Job drawing, mm, ordinate dimensions from the low corner. One solid piece. Give positions to 0.01 mm unless a question says otherwise; leave off trailing zeros. Order: outer loops, then holes, each group sorted by start corner. A loop starts at its lowest first (then second) coordinate and runs counter-clockwise, first axis right, second up. Notation, with made-up numbers: M -32,-3.75 L 18,-3.75 A30 cw 18,25.25 Z; hole C 56.25,56.25 d4. An arc over 180 degrees is marked long. Use CSV: the item, a comma, the result in double quotes. Start each with the question number.
Item 1: Two-plate mould, pull along X, no slides. Class the marked faces 1, 2 and 3: pulls with the +X half, pulls with the -X half, needs draft (parallel to the pull), parting line crosses it, or undercut.
Item 2: Band-saw the part on B-B on y = 30. Write the cut outline in (x, z).
Item 3: Wall check: line 1 along Y through (x, z) = (30, 22); line 2 along X through (y, z) = (30.5, 27); line 3 along X through (y, z) = (39, 14). Give the ranges that are in metal, low to high.
Item 4: Pin check, flat tips, straight feed: P1, Ø10, axis at y = 49, z = 7.5, coming from the +X side; P2, Ø6, axis at x = 29.5, z = 23.5, coming from the +Y side; P3, Ø6, axis at x = 52, z = 5, coming from the +Y side; P4, Ø1.5, axis at x = 50.5, y = 53.5, coming from the -Z side. Stop position of each tip, or through.
Item 5: Band-saw the part on A-A on x = 30. Write the cut outline in (y, z), plus the area to 3 significant figures.
Item 6: Band-saw the part on C-C on z = 38.5. Write the cut outline in (x, y).
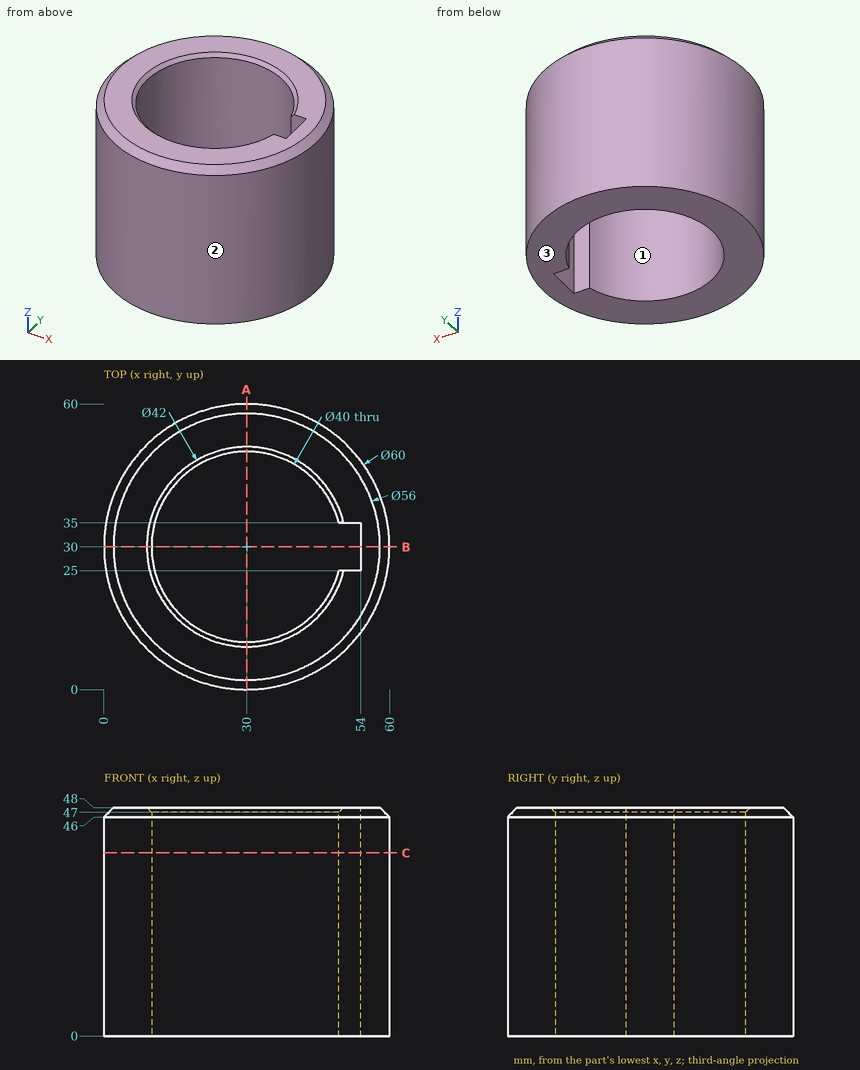
Model answer:
1,face 1,"undercut"
1,face 2,"parting line crosses it"
1,face 3,"needs draft"
2,outline,"M 0,0 L 10,0 L 10,47 L 9,48 L 2,48 L 0,46 Z; M 54,0 L 60,0 L 60,46 L 58,48 L 54,48 Z"
3,line 1,"y = 0 to 10, 50 to 60"
3,line 2,"x = 0 to 10.01, 54 to 60"
3,line 3,"x = 1.38 to 12.14, 47.86 to 58.62"
4,P1,"stops at x = 56.53"
4,P2,"stops at y = 60"
4,P3,"stops at y = 53.22"
4,P4,"passes through"
5,outline,"M 0,0 L 10,0 L 10,47 L 9,48 L 2,48 L 0,46 Z; M 50,0 L 60,0 L 60,46 L 58,48 L 51,48 L 50,47 Z"
5,area,"955 mm^2"
6,outline,"C 30,30 d60; hole M 49.36,25 L 54,25 L 54,35 L 49.36,35 A20 ccw long Z"
